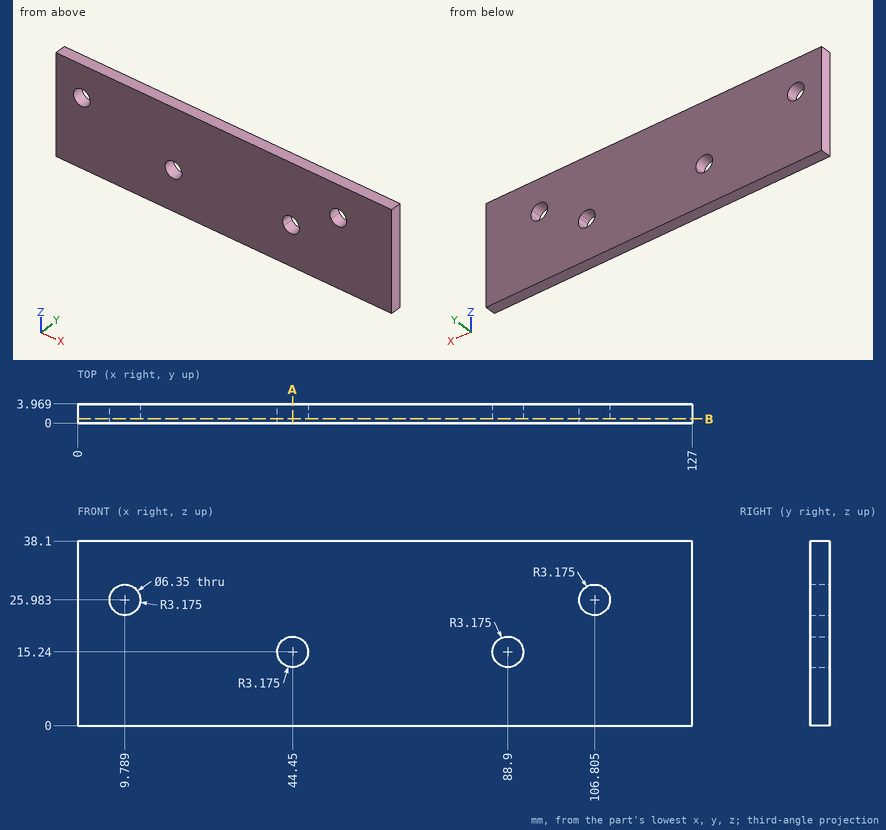
The figure shows three views and two pictorial views of one solid part (mm, origin at its lowest corner). Answer the questions. Coordinates: 2 decimals unless noted, no trailing zeros. Order: outer loops, then holes, each group sorted by start corner. A loop starts at its lowest first (then second) coordinate and runs counter-clockwise, first axis right, second up.
Q1. Consider line 1 (X direction, y = 1.45, z = 28) (1 decimal); line 2 (Z direction, x = 89, y = 3); line 3 (Z direction, x = 107, y = 2.65) (1 decimal). Determine where each line is inside the solid, lowest interval first.
Q2. Given P1, Ø10, axis at x = 9.79, z = 25.98, coming from the +Y side, flat-ended and moving along its own axis, determine where the tip first touches the part or whether it passes through.
Q3. A cutting plane is placed at B-B, the plane y = 0.9. State how many separate pieces and enclosed holes the cut face has, and give its area (3 significant figures).
Q4. A cutting plane is placed at A-A, the plane x = 44.45. Write down the section's boundary in (y, z) (1 decimal), and give its area (3 significant figures).
Answers follow:
1. line 1: x = 0 to 7.3, 12.2 to 104.4, 109.3 to 127
1. line 2: z = 0 to 12.07, 18.41 to 38.1
1. line 3: z = 0 to 22.8, 29.2 to 38.1
2. P1: stops at y = 3.97
3. separate pieces: 1
3. enclosed holes: 4
3. area: 4,710 mm2
4. outline: (0, 0) - (4, 0) - (4, 12.1) - (0, 12.1) - close; (0, 18.4) - (4, 18.4) - (4, 38.1) - (0, 38.1) - close
4. area: 126 mm2
